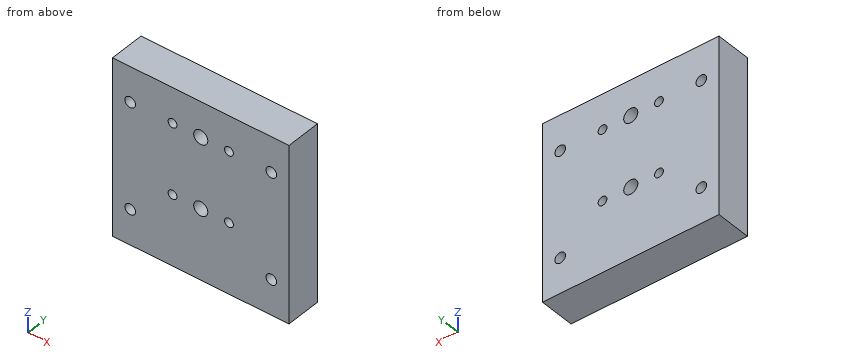
```python
from build123d import *

# Parameters (mm, degrees)
SKETCH_1_W          = 100
SKETCH_1_H          = 100
EXTRUDE_1_DEPTH     = 20
SKETCH_2_R          = 3
SKETCH_2_R_2        = 2.5
SKETCH_2_R_3        = 4
CUT_EXTRUDE_1_DEPTH = 20


with BuildPart() as part:
    # Эскиз1 → Бобышка-Вытянуть1 (new body)
    with BuildSketch(Plane(origin=(0, 0, 0), x_dir=(1, 0, 0), z_dir=(0, 1, 0))):
        with Locations((50, 50)):
            Rectangle(SKETCH_1_W, SKETCH_1_H)
    extrude(amount=EXTRUDE_1_DEPTH)

    # Эскиз2 → Вырез-Вытянуть1 (cut)
    with BuildSketch(Plane(origin=(0, 20, 0), x_dir=(1, 0, 0), z_dir=(0, 1, 0))):
        with Locations(Location((10, 80, 0), (0, 0, 270))):
            Circle(SKETCH_2_R)
        with Locations(Location((90, 80, 0), (0, 0, 270))):
            Circle(SKETCH_2_R)
        with Locations(Location((34, 60, 0), (0, 0, 270))):
            Circle(SKETCH_2_R_2)
        with Locations(Location((50, 20, 0), (0, 0, 270))):
            Circle(SKETCH_2_R_3)
        with Locations(Location((66, 60, 0), (0, 0, 270))):
            Circle(SKETCH_2_R_2)
        with Locations(Location((10, 20, 0), (0, 0, 270))):
            Circle(SKETCH_2_R)
        with Locations(Location((50, 60, 0), (0, 0, 270))):
            Circle(SKETCH_2_R_3)
        with Locations(Location((90, 20, 0), (0, 0, 270))):
            Circle(SKETCH_2_R)
        with Locations(Location((34, 20, 0), (0, 0, 270))):
            Circle(SKETCH_2_R_2)
        with Locations(Location((66, 20, 0), (0, 0, 270))):
            Circle(SKETCH_2_R_2)
    extrude(amount=-CUT_EXTRUDE_1_DEPTH, mode=Mode.SUBTRACT)


solid = part.part
```
Design review of the part built by this model. Coordinates are the model's own, in mm. Coordinates: 2 decimals unless noted, no trailing zeros. Write each loop counter-clockwise with the first axis right and the second up, starting at its lowest first coordinate (ties: lowest second). Pieces come first, ordered by that corner, then holes.
1) Add section B-B (y = 8.75). State how many separate pieces and enclosed holes the cut face has, plus the area to 3 significant figures.
2) Add section D-D (x = 10). Write out the cut boundary in (y, z).
3) Add section A-A (x = 34). Write out the cut boundary in (y, z).
4) To check wall thickness, follow L1, parallel to X at y = 4.25, z = -20; L2, parallel to X at y = 15.25, z = -60; L3, parallel to X at y = 16.25, z = -19.5. State the ranges of each line that lie inside material, in increasing order.
5) Add section C-C (z = -60). Write out the cut boundary in (x, y), plus the area to 3 significant figures.
Check result:
1. separate pieces: 1
1. enclosed holes: 10
1. area: 9,710 mm2
2. outline: (0, -100) - (20, -100) - (20, -83) - (0, -83) - close; (0, -77) - (20, -77) - (20, -23) - (0, -23) - close; (0, -17) - (20, -17) - (20, 0) - (0, 0) - close
3. outline: (0, -100) - (20, -100) - (20, -62.5) - (0, -62.5) - close; (0, -57.5) - (20, -57.5) - (20, -22.5) - (0, -22.5) - close; (0, -17.5) - (20, -17.5) - (20, 0) - (0, 0) - close
4. L1: x = 0 to 7, 13 to 31.5, 36.5 to 46, 54 to 63.5, 68.5 to 87, 93 to 100
4. L2: x = 0 to 31.5, 36.5 to 46, 54 to 63.5, 68.5 to 100
4. L3: x = 0 to 7.04, 12.96 to 31.55, 36.45 to 46.03, 53.97 to 63.55, 68.45 to 87.04, 92.96 to 100
5. outline: (0, 0) - (31.5, 0) - (31.5, 20) - (0, 20) - close; (36.5, 0) - (46, 0) - (46, 20) - (36.5, 20) - close; (54, 0) - (63.5, 0) - (63.5, 20) - (54, 20) - close; (68.5, 0) - (100, 0) - (100, 20) - (68.5, 20) - close
5. area: 1,640 mm2
